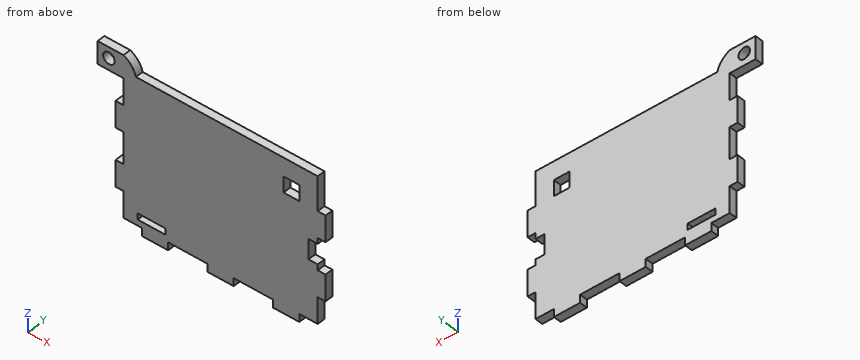
Autodesk Inventor part; units mm, degrees
ref_plane "YZ Plane" through (0, 0, 0) normal (1, 0, 0) x (0, 1, 0)
ref_plane "XZ Plane" through (0, 0, 0) normal (0, 1, 0) x (-1, 0, 0)
ref_plane "XY Plane" through (0, 0, 0) normal (0, 0, 1) x (1, 0, 0)
sketch "Esboço1" plane through (0, 0, 0) normal (0, 1, 0) x (-1, 0, 0)
  line L0 (0, 0) -> (-74, 0)
  line L1 (-74, 0) -> (-74, -52)
  line L2 (-74, -52) -> (0, -52)
  line L3 (0, -52) -> (0, 0)
  line L4 (-6.0465, -39.0348) -> (-22.7965, -39.0348)
  line L5 (-22.7965, -39.0348) -> (-22.7965, -36.6698)
  line L6 (-22.7965, -36.6698) -> (-6.0465, -36.6698)
  line L7 (-6.0465, -36.6698) -> (-6.0465, -39.0348)
  dimension "d0" = 74
  dimension "d1" = 52
  dimension "d22" = 16.75
  dimension "d23" = 2.365
extrude "Extrusão1" add sketch "Esboço1" along normal blind 3 contours L3 L2 L1 L0 | L4 L5 L6 L7
sketch "Esboço2" plane through (0, 3, 0) normal (0, 1, 0) x (1, 0, 0)
  line L0 (0, 0) -> (74, 0)
  line L1 (0, 52) -> (0, 0)
  line L2 (74, 52) -> (0, 52)
  line L3 (7, 52) -> (17, 52)
  line L4 (17, 52) -> (17, 55)
  line L5 (17, 55) -> (7, 55)
  line L6 (7, 55) -> (7, 52)
  line L7 (32, 52) -> (42, 52)
  line L8 (42, 52) -> (42, 55)
  line L9 (42, 55) -> (32, 55)
  line L10 (32, 55) -> (32, 52)
  line L11 (57, 52) -> (67, 52)
  line L12 (67, 52) -> (67, 55)
  line L13 (67, 55) -> (57, 55)
  line L14 (57, 55) -> (57, 52)
  line L15 (74, 0) -> (74, 52)
  point P0 (17, 52)
  point P1 (67, 52)
  point P2 (42, 52)
  point P3 (74, 26)
  point P4 (32, 53.5)
  point P5 (17, 53.5)
  point P6 (7, 53.5)
  point P7 (67, 53.5)
  point P8 (42, 53.5)
  point P9 (57, 53.5)
  dimension "d13" = 3
  dimension "d40" = 7
  dimension "d41" = 7
  dimension "d43" = 10
  dimension "d46" = 10
  dimension "d52" = 10
  dimension "d54" = 40
  dimension "d55" = 15
extrude "Extrusão2" add sketch "Esboço2" against normal blind 3 contours L6 L5 L4 L2 | L2 L14 L13 L12 | L10 L9 L8 L2
sketch "Esboço4" plane through (0, 0, 0) normal (0, -1, 0) x (1, 0, 0)
  line L0 (16.0248, -49.74) -> (5.3998, -49.74)
  line L1 (5.3998, -49.74) -> (5.3998, -47.39)
  line L2 (5.3998, -47.39) -> (16.0248, -47.39)
  line L3 (16.0248, -47.39) -> (16.0248, -49.74)
  line L4 (7, -52) -> (0, -52)
  point P0 (0, 0)
  dimension "d24" = 10.625
  dimension "d25" = 2.35
  dimension "d120" = 2.26
extrude "Extrusão3" cut sketch "Esboço4" against normal blind 3
sketch "Esboço5" plane through (0, 3, 0) normal (0, 1, 0) x (1, 0, 0)
  line L0 (70.5, 22.2) -> (74, 22.2)
  line L1 (74, 22.2) -> (74, 29.8)
  line L2 (74, 29.8) -> (70.5, 29.8)
  line L3 (70.5, 29.8) -> (70.5, 22.2)
  line L4 (74, 0) -> (74, 52)
  line L5 (74, 52) -> (67, 52)
  point P0 (0, 0)
  point P1 (74, 26)
  point P2 (72.25, 29.8)
  dimension "d47" = 3.5
  dimension "d48" = 7.6
  dimension "d51" = 0
  dimension "d79" = 22.2
extrude "Extrusão4" cut sketch "Esboço5" against normal blind 10
sketch "Esboço6" plane through (0, 3, 0) normal (0, 1, 0) x (1, 0, 0)
  line L0 (0, 10) -> (-3, 10)
  line L1 (-3, 10) -> (-3, 20)
  line L2 (-3, 20) -> (0, 20)
  line L3 (0, 20) -> (0, 10)
  line L4 (0, 32) -> (-3, 32)
  line L5 (-3, 32) -> (-3, 42)
  line L6 (-3, 42) -> (0, 42)
  line L7 (0, 42) -> (0, 32)
  line L8 (7, 52) -> (0, 52)
  line L9 (0, 0) -> (74, 0)
  line L10 (74, 52) -> (67, 52)
  line L11 (0, 0) -> (74, 0)
  line L12 (74, 0) -> (74, 22.2)
  line L13 (74, 10) -> (77, 10)
  line L14 (77, 10) -> (77, 20)
  line L15 (77, 20) -> (74, 20)
  line L16 (74, 20) -> (74, 10)
  line L17 (74, 29.8) -> (74, 52)
  line L18 (74, 32) -> (77, 32)
  line L19 (77, 32) -> (77, 42)
  line L20 (77, 42) -> (74, 42)
  line L21 (74, 42) -> (74, 32)
  point P0 (-1.5, 42)
  point P1 (7, 0)
  point P2 (-1.5, 10)
  point P3 (67, 0)
  point P4 (75.5, 10)
  dimension "d62" = 3
  dimension "d63" = 10
  dimension "d64" = 3
  dimension "d65" = 10
  dimension "d66" = 10
  dimension "d67" = 10
  dimension "d74" = 3
  dimension "d75" = 10
  dimension "d76" = 10
extrude "Extrusão5" add sketch "Esboço6" against normal blind 3
sketch "Esboço8" plane through (0, 0, 0) normal (0, -1, 0) x (1, 0, 0)
  line L0 (0, 0) -> (74, 0)
  line L1 (4.9609, 0) -> (-9.8465, 0)
  line L2 (-9.8465, 0) -> (-9.8465, 8.6)
  line L3 (0, -10) -> (0, 0)
  circle A0 centre (-5.5465, 4.4971) radius 2.2
  line L4 (-9.8465, 8.6) -> (0, 8.6)
  line L5 (0, 8.6) -> (0, 0)
  line L6 (0, 0) -> (-9.8465, 0)
  line L7 (-9.8465, 0) -> (-9.8465, 8.6)
  arc A1 (4.9609, 0) -> (0, 8.6) centre (-3.4963, 0.8523) ccw
  point P0 (0, 4.3)
  point P1 (-4.9233, 8.6)
  dimension "d100" = 8.6
  dimension "d102" = 4.4
  dimension "d104" = 4.3
  dimension "d121" = 8.5
  dimension "d123" = 4.15
  dimension "d124" = 5.55
  dimension "d128" = 9.8465
  dimension "d130" = 9.8465
extrude "Extrusão7" add sketch "Esboço8" against normal blind 3
sketch "Esboço11" plane through (0, 0, 0) normal (0, -1, 0) x (1, 0, 0)
  line L0 (0, 0) -> (74, 0)
  line L1 (74, 0) -> (74, 3)
  line L2 (74, 3) -> (0, 3)
  line L3 (0, 3) -> (0, 0)
  dimension "d129" = 3
extrude "Extrusão9" add sketch "Esboço11" against normal blind 3
sketch "Esboço12" plane through (0, 3, 0) normal (0, 1, 0) x (1, 0, 0)
  line L0 (67, 4) -> (61, 4)
  line L1 (61, 4) -> (61, 10)
  line L2 (61, 10) -> (67, 10)
  line L3 (67, 10) -> (67, 4)
  line L4 (4.728, -3) -> (74, -3)
  line L5 (74, -3) -> (74, 10)
  line L6 (74, 10) -> (77, 10)
  point P0 (0, 0)
  point P1 (64, 4)
  point P2 (67, 7)
  point P3 (75.5, 10)
  dimension "d131" = 6
  dimension "d132" = 6
  dimension "d134" = 7
  dimension "d135" = 0
extrude "Extrusão10" cut sketch "Esboço12" against normal blind 10
properties part number "Parede_HX711"
Work out the finished part from the listing and answer in its coordinate system (mm). Round coordinates to 2 decimals unless told otherwise and drop trailing zeros. Write each loop counter-clockwise with the first axis right and the second up, starting at its lowest first coordinate (ties: lowest second). Pieces come first, ordered by that corner, then holes.
1) A cutting plane is placed at B-B (x = 40). Give the vertices of the cut face in (y, z).
2) A cutting plane is placed at D-D (y = 1.5). Give the number of separate pieces and of enclosed holes in the cut face, plus the area to 3 significant figures.
3) Straight lines are drawn through the part: line 1 (Z direction, x = 61.5, y = 2.3); line 2 (Z direction, x = 14, y = 0.8); line 3 (X direction, y = 0.9, z = -49). For each, find the intervals that lie inside material, in ascending order.
4) A cutting plane is placed at A-A (x = 11.5). Give the vertices of the cut face in (y, z), plus the area to 3 significant figures.
5) A cutting plane is placed at C-C (z = -36). Give the vertices of the cut face in (x, y).
6) Given pin 1 Ø0.9 at (y, z) = (1, -53) entering from -X; pin 2 Ø1.2 at (y, z) = (1.5, -48.5) entering from +X; pin 3 Ø1.5 at (y, z) = (2, -53) entering from +X, each flat-ended and moving along its own axis, determine where each tip first touches the part or whether it passes through.
Completed:
1. outline: (0, -55) - (3, -55) - (3, 3) - (0, 3) - close
2. separate pieces: 1
2. enclosed holes: 3
2. area: 4,280 mm2
3. line 1: z = -55 to -10, -4 to 3
3. line 2: z = -55 to -49.74, -47.39 to 3
3. line 3: x = 0 to 5.4, 16.02 to 74
4. outline: (0, -55) - (3, -55) - (3, -49.74) - (0, -49.74) - close; (0, -47.39) - (3, -47.39) - (3, 3) - (0, 3) - close
4. area: 167 mm2
5. outline: (-3, 0) - (77, 0) - (77, 3) - (-3, 3) - close
6. pin 1: stops at x = 7
6. pin 2: stops at x = 74
6. pin 3: stops at x = 67
